Design review of the part built by this model. Coordinates are the model's own, in mm. A direction names the side the tool comes from. Coordinates: 2 decimals unless noted, no trailing zeros. Put each result on its own line as item: value. Start each with the question number.
(1) Clearance check with flat-ended pins moving along their axes: pin 1 (6 mm diameter, centred on x = 29.5, z = 3, fed in from -Y) (3 decimals); pin 2 (11 mm diameter, centred on y = 35, z = 1, fed in from +X); pin 3 (2 mm diameter, centred on x = 30, y = 38, fed in from +Z); pin 4 (5 mm diameter, centred on x = 36, z = 9.5, fed in from -Y). State where each tip first meets the part, or that it passes through.
(2) For probe 1 along Y at (x, z) = (34.5, 0); probe 2 along X at (y, z) = (21.5, 6); probe 3 along Z at (x, y) = (34.5, 36), list the stretches that pass through material, from the lowest coordinate up. Write a range as [from, to].
(3) The part is to be moulded in two halves that separate along Y. For faces 1 (the flat face through (39.746, 37, 6)), 2 (the cylindrical face through (33.57, 31.91, -1.03)), 3 (the cylindrical face through (33.603, 17.528, -0.838)), say which applies: +Y half, -Y half, draft (parallel to the pull), parting line (faces both ways), or undercut.
(4) For faces 4 (the flat face through (27.554, 42, 0)), 5 (the cylindrical face through (38.35, 33.46, 13.96)), 6 (the cylindrical face through (28.93, 22.3, -0.63)), list the 3-axis set-ups (+Z, -Z, +X, -X, +Y, -Y) from which the entire face can be reached by the end or side of a thin tool; tool diameter is ignored.
```python
from build123d import *

# Parameters (mm, degrees)
SKETCH3_R          = 4.7625
CUT_EXTRUDE1_DEPTH = 13.192
CHAMFER1_SIZE      = 0.508


with BuildPart() as part:
    # Sketch2 → Revolve1 (revolve)
    with BuildSketch(Plane.XY):
        with BuildLine():
            Line((27.553988289, 50.300658572), (27.553988289, 36.559258572))
            Line((27.553988289, 36.559258572), (33.638296362, 36.559258572))
            Line((33.638296362, 36.559258572), (39.745988289, 36.571958572))
            Line((39.745988289, 36.571958572), (39.745988289, 50.351458572))
            Line((39.745988289, 50.351458572), (39.237988289, 50.859458572))
            Line((39.237988289, 50.859458572), (37.483216953, 50.859458572))
            ThreePointArc((37.483216953, 50.859458572), (36.944383174, 51.073319594), (36.697988289, 51.598074717))
            Line((36.697988289, 51.598074717), (36.697988289, 55.077874717))
            Line((36.697988289, 55.077874717), (36.166604435, 55.609258572))
            Line((36.166604435, 55.609258572), (31.109988289, 55.609258572))
            Line((31.109988289, 55.609258572), (30.601988289, 55.101258572))
            Line((30.601988289, 55.101258572), (30.601988289, 51.621458572))
            ThreePointArc((30.601988289, 51.621458572), (30.371364168, 51.064682692), (29.814588289, 50.834058572))
            Line((29.814588289, 50.834058572), (28.061988289, 50.834058572))
            Line((28.061988289, 50.834058572), (27.553988289, 50.300658572))
        make_face()
    revolve(axis=Axis((33.638296362, 36.559258572, 0), (-1, 0, 0)))

    # Sketch3 → Cut-Extrude1 (cut, through all)
    with BuildSketch(Plane.ZY.offset(-27.553988289)):
        with Locations((0, 36.559258572)):
            Circle(SKETCH3_R)
    extrude(amount=-CUT_EXTRUDE1_DEPTH, mode=Mode.SUBTRACT)

    # Chamfer1
    chamfer1_edges = [part.edges().sort_by_distance(p)[0] for p in [
        (39.745988289, 36.559258572, -4.7625),
        (27.553988289, 36.559258572, -4.7625),
    ]]
    chamfer(chamfer1_edges, length=CHAMFER1_SIZE)


solid = part.part
```
Computed values:
1. pin 1: stops at y = 17.515
1. pin 2: stops at x = 39.75
1. pin 3: stops at z = 18.89
1. pin 4: stops at y = 18.84
2. probe 1: y = [17.51, 31.8], [41.32, 55.61]
2. probe 2: x = [30.6, 36.7]
2. probe 3: z = [-19.04, -4.73], [4.73, 19.04]
3. face 1: draft
3. face 2: undercut
3. face 3: parting line
4. face 4: +Z, -Z, -X, +Y, -Y
4. face 5: +X
4. face 6: -X
